Autodesk Inventor part; units mm, degrees
ref_plane "YZ Plane" through (0, 0, 0) normal (1, 0, 0) x (0, 1, 0)
ref_plane "XZ Plane" through (0, 0, 0) normal (0, 1, 0) x (-1, 0, 0)
ref_plane "XY Plane" through (0, 0, 0) normal (0, 0, 1) x (1, 0, 0)
sketch "Esboço1" plane through (0, 0, 0) normal (0, 0, 1) x (1, 0, 0)
  line L0 (0, 0) -> (50, 0)
  line L1 (50, 0) -> (50, -31.4)
  line L2 (50, -31.4) -> (0, -31.4)
  line L3 (0, -31.4) -> (0, 0)
  dimension "d0" = 50
  dimension "d1" = 31.4
extrude "Extrusão1" add sketch "Esboço1" along normal blind 0.5
sketch "Esboço2" plane through (0, 0, 0.5) normal (0, 0, 1) x (1, 0, 0)
  line L0 (0, -31.4) -> (50, -31.4)
  line L1 (50, -31.4) -> (43.6, -31.4)
  line L2 (43.6, -31.4) -> (43.6, 0)
  line L3 (50, 0) -> (0, 0)
  line L4 (43.6, 0) -> (50, 0)
  line L5 (50, -31.4) -> (50, 0)
  line L6 (50, 0) -> (50, -31.4)
  dimension "d4" = 6.4
extrude "Extrusão2" cut sketch "Esboço2" against normal blind 0.5
sketch "Esboço3" plane through (0, 0, 0.5) normal (0, 0, 1) x (1, 0, 0)
  line L0 (0, -31.4) -> (43.6, -31.4)
  line L1 (43.6, -31.4) -> (13.6, -31.4)
  line L2 (13.6, -31.4) -> (13.6, -34.4)
  line L3 (13.6, -34.4) -> (43.6, -34.4)
  line L4 (43.6, -34.4) -> (43.6, -31.4)
  point P0 (0, 0)
  dimension "d7" = 30
  dimension "d8" = 3
extrude "Extrusão3" add sketch "Esboço3" against normal blind 0.5
sketch "Esboço4" plane through (0, 0, 0.5) normal (0, 0, 1) x (1, 0, 0)
  line L0 (43.6, -34.4) -> (43.6, 0)
  line L1 (43.6, -34.4) -> (44.6, -34.4)
  line L2 (44.6, -34.4) -> (44.6, 0)
  line L3 (44.6, 0) -> (43.6, 0)
  line L4 (43.6, 0) -> (43.6, -34.4)
  point P0 (0, 0)
  dimension "d11" = 1
extrude "Extrusão4" add sketch "Esboço4" against normal blind 0.5
sketch "Esboço5" plane through (0, 0, 0.5) normal (0, 0, 1) x (1, 0, 0)
  line L0 (44.6, -34.4) -> (13.6, -34.4)
  line L1 (44.6, -34.4) -> (44.6, -29.5)
  line L2 (44.6, 0) -> (44.6, -34.4)
  line L3 (44.6, 0) -> (44.6, -7.4)
  line L4 (44.6, -7.4) -> (29.6, -7.4)
  line L5 (44.6, -29.5) -> (29.6, -29.5)
  line L6 (29.6, -29.5) -> (29.6, -30.5)
  line L7 (29.6, -30.5) -> (44.6, -30.5)
  line L8 (29.6, -7.4) -> (29.6, -6.4)
  line L9 (29.6, -6.4) -> (44.6, -6.4)
  line L10 (44.6, -7.4) -> (44.6, -6.4)
  line L11 (29.6, -6.4) -> (30.1, -6.4)
  line L12 (30.1, -6.4) -> (30.1, 0)
  line L13 (44.6, 0) -> (0, 0)
  line L14 (29.6, 0) -> (29.6, -6.4)
  line L15 (29.6, -30.5) -> (29.6, -34.4)
  line L16 (30.1, -30.5) -> (30.1, -34.4)
  line L17 (29.6, -34.4) -> (30.1, -34.4)
  dimension "d14" = 4.9
  dimension "d15" = 7.4
  dimension "d16" = 15
  dimension "d17" = 15
  dimension "d18" = 1
  dimension "d19" = 1
  dimension "d20" = 0.5
extrude "Extrusão5" add sketch "Esboço5" along normal blind 12 contours L0 L15 L7 L16 | L7 L6 L5 L1 | L2 L4 L8 L9 | L12 L9 L14 L13
sketch "Esboço6" plane through (0, 0, 0.5) normal (0, 0, 1) x (1, 0, 0)
  line L0 (44.6, -34.4) -> (44.6, -30.5)
  line L1 (44.6, -34.4) -> (45.6, -34.4)
  line L2 (45.6, -34.4) -> (45.6, 0)
  line L3 (45.6, 0) -> (44.6, 0)
  line L4 (44.6, 0) -> (44.6, -34.4)
  point P0 (0, 0)
  dimension "d23" = 1
extrude "Extrusão6" add sketch "Esboço6" against normal blind 0.5
sketch "Esboço7" plane through (0, 0, 0.5) normal (0, 0, 1) x (1, 0, 0)
  line L0 (44.6, -30.5) -> (30.1, -30.5)
  line L1 (44.6, -30.5) -> (45.6, -30.5)
  line L2 (45.6, -34.4) -> (45.6, 0)
  line L3 (45.6, -30.5) -> (45.6, -6.4)
  line L4 (30.1, -6.4) -> (44.6, -6.4)
  line L5 (44.6, -6.4) -> (45.6, -6.4)
  line L6 (44.6, -6.4) -> (44.6, -30.5)
  point P0 (0, 0)
extrude "Extrusão7" add sketch "Esboço7" along normal blind 12
sketch "Esboço8" plane through (0, 0, 0.5) normal (0, 0, 1) x (1, 0, 0)
  line L0 (29.6, -29.5) -> (29.6, -34.4)
  line L1 (29.6, -31.7209) -> (18.1, -31.7209)
  line L2 (18.1, -34.4) -> (18.1, -31.7209)
  line L3 (18.1, -31.7209) -> (18.1, -12.7)
  line L4 (18.1, -12.7) -> (0, -12.7)
  line L5 (0, 0) -> (0, -31.4)
  line L6 (18.1, -34.4) -> (0, -34.4)
  line L7 (0, -34.4) -> (0, -12.7)
  dimension "d28" = 11.5
extrude "Extrusão8" cut sketch "Esboço8" against normal blind 12
sketch "Esboço9" plane through (0, 0, 0.5) normal (0, 0, 1) x (1, 0, 0)
  line L0 (0, 0) -> (0, -12.7)
  line L1 (0, 0) -> (-5, 0)
  line L2 (-5, 0) -> (-5, -12.7)
  line L3 (-5, -12.7) -> (0, -12.7)
  line L4 (0, -12.7) -> (0, 0)
  dimension "d31" = 5
extrude "Extrusão9" add sketch "Esboço9" against normal blind 12
fillet "Arredondamento1" radius 10 1 edges at (-5, -6.35, -11.5)
sketch "Esboço10" plane through (0, 0, 0.5) normal (0, 0, 1) x (1, 0, 0)
  line L0 (-5, 0) -> (-5, -12.7)
  line L1 (-5, 0) -> (22, 0)
  line L2 (22, 0) -> (22, -12.7)
  line L3 (22, -12.7) -> (-5, -12.7)
  line L4 (-5, -12.7) -> (-5, 0)
  point P0 (0, 0)
  dimension "d37" = 27
extrude "Extrusão10" add sketch "Esboço10" along normal blind 1
sketch "Esboço11" plane through (30.1, -6.4, 0.5) normal (1, 0, 0) x (0, 0, -1)
  line L0 (0, 6.4) -> (-12, 6.4)
  line L1 (-12, 6.4) -> (-6, 6.4)
  line L2 (-6, 6.4) -> (-6, -28)
  line L3 (0, -28) -> (-12, -28)
  line L4 (-6, 6.4) -> (-6, 3.2)
  line L5 (-6, -28) -> (-6, -26.1)
  circle A0 centre (-6, -26.1) radius 0.5
  circle A1 centre (-6, 3.2) radius 0.5
  point P0 (0.5, 6.4)
  dimension "d38" = 3.2
  dimension "d39" = 1.9
  dimension "d40" = 1
  dimension "d41" = 1
extrude "Extrusão11" cut sketch "Esboço11" against normal blind 1
properties part number "tampa 2"
For this review, take the finished solid that the model builds, in its own axes (mm). A direction names the side the tool comes from. Round coordinates to 2 decimals unless told otherwise and drop trailing zeros. Write each loop counter-clockwise with the first axis right and the second up, starting at its lowest first coordinate (ties: lowest second). Pieces come first, ordered by that corner, then holes. Notation, with made-up numbers: (8, 63) - (33, 63) arc R25 ccw to (33, 76) - close; hole circle Ø8 at (66.5, 81.25). An arc over 180 degrees is marked (long way). Use a Markdown table: item, result.
Q1. The part is to be moulded in two halves that separate along Y. For faces 6 (the flat face through (38, -6.4, 6)), 7 (the flat face through (45.6, -17, 6)), 8 (the flat face through (44.6, -18, 6)), say which applies: pulls with the +Y half, pulls with the -Y half, needs draft (parallel to the pull), parting line crosses it, or undercut.
Derived:
| item | result |
|---|---|
| face 6 | pulls with the +Y half |
| face 7 | needs draft |
| face 8 | undercut |
Q2. We need section C-C (x = 32.5). Give the boundary of the cut face in (y, z), plus the area to 3 significant figures.
Derived:
| item | result |
|---|---|
| outline | (-34.4, 0) - (0, 0) - (0, 0.5) - (-6.4, 0.5) - (-6.4, 12.5) - (-7.4, 12.5) - (-7.4, 0.5) - (-29.5, 0.5) - (-29.5, 12.5) - (-30.5, 12.5) - (-30.5, 0.5) - (-34.4, 0.5) - close |
| area | 41.2 mm2 |
Q3. Wall thickness on line 1 along Y through (x, z) = (29.9, 6.5); line 2 along X through (y, z) = (-11.5, 4.25); line 3 along X through (y, z) = (-5, 9): over which ranges is each line inside the solid? List them lowest first.
Derived:
| item | result |
|---|---|
| line 1 | y = -34.4 to -33, -32 to -29.5, -7.4 to -3.7, -2.7 to 0 |
| line 2 | x = 44.6 to 45.6 |
| line 3 | x = 29.6 to 30.1 |
Q4. We need section B-B (y = -21). Give the boundary of the cut face in (x, z).
Derived:
| item | result |
|---|---|
| outline | (18.1, 0) - (45.6, 0) - (45.6, 12.5) - (44.6, 12.5) - (44.6, 0.5) - (18.1, 0.5) - close |
Q5. We need section A-A (z = 3.25). Give the boundary of the cut face in (x, y), plus the area to 4 significant figures.
Derived:
| item | result |
|---|---|
| outline | (29.6, -34.4) - (30.1, -34.4) - (30.1, -30.5) - (45.6, -30.5) - (45.6, -6.4) - (30.1, -6.4) - (30.1, 0) - (29.6, 0) - (29.6, -7.4) - (44.6, -7.4) - (44.6, -29.5) - (29.6, -29.5) - close |
| area | 59.25 mm2 |
Q6. Clearance check with flat-ended pins moving along their axes: pin 1 (9.5 mm diameter, centred on x = 37, z = 9, fed in from +Y); pin 2 (2.5 mm diameter, centred on y = -32, z = 7, fed in from -X); pin 3 (10 mm diameter, centred on x = 31, y = -16, fed in from +Z). State where each tip first meets the part, or that it passes through.
Derived:
| item | result |
|---|---|
| pin 1 | stops at y = -6.4 |
| pin 2 | stops at x = 29.6 |
| pin 3 | stops at z = 0.5 |
Q7. Machinability: for faces 1 (the flat face through (0, -6, -6)), 2 (the flat face through (37, -29.5, 6)), 3 (the flat face through (38, -32, 0.5)), 4 (the flat face through (22, -6, 1)), 5 (the flat face through (30.1, -4, 6)), which of the approach directions +Z, -Z, +X, -X, +Y, -Y give a long, thin tool a straight path to every point of the face, cutting with its end or side? Answer none if there is none.
Derived:
| item | result |
|---|---|
| face 1 | -Z, +X, +Y, -Y |
| face 2 | +Z, -X |
| face 3 | +Z, +X, -Y |
| face 4 | +Z, +Y, -Y |
| face 5 | +Z, +X, +Y |
Q8. We need section D-D (y = -8). Give the boundary of the cut face in (x, z).
Derived:
| item | result |
|---|---|
| outline | (-5, -2.84) arc R10 ccw to (0, -11.5) - (0, 0) - (45.6, 0) - (45.6, 12.5) - (44.6, 12.5) - (44.6, 0.5) - (22, 0.5) - (22, 1.5) - (-5, 1.5) - close |
